Verification items for the finished model (mm, model axes). A direction names the side the tool comes from. Round coordinates to 2 decimals unless told otherwise and drop trailing zeros. Order: outer loops, then holes, each group sorted by start corner. A loop starts at its lowest first (then second) coordinate and runs counter-clockwise, first axis right, second up. Notation, with made-up numbers: M 77,23 L 118,23 A24 cw 118,34 Z; hole C 8,82 d5. An arc over 180 degrees is marked long. Return JSON: item names as keys, results as strings. Group by question number.
from build123d import *

# Parameters (mm, degrees)
SKETCH_W        = 63.5
SKETCH_H        = 21
PAD_DEPTH       = 25
SKETCH001_W     = 63
SKETCH001_H     = 21
POCKET_DEPTH    = 25
SKETCH006_W     = 8
SKETCH006_H     = 6
SKETCH006_H_2   = 2.5
POCKET004_DEPTH = 5
SKETCH007_R     = 0.7
POCKET005_DEPTH = 5
CHAMFER_SIZE    = 0.6


with BuildPart() as part:
    # Sketch → Pad (new body)
    with BuildSketch(Plane.XY):
        with Locations((31.75, 10.5)):
            Rectangle(SKETCH_W, SKETCH_H)
    extrude(amount=PAD_DEPTH)

    # Sketch001 (on Face6 of Pad) → Pocket (cut)
    with BuildSketch(Plane.XY.offset(25)):
        with Locations((32.5, 10.5)):
            Rectangle(SKETCH001_W, SKETCH001_H)
    extrude(amount=-POCKET_DEPTH, mode=Mode.SUBTRACT)

    # Sketch006 → Pocket004 (cut)
    with BuildSketch(Plane(origin=(0, 0, 0), x_dir=(0, -1, 0), z_dir=(-1, 0, 0))):
        with Locations((-10.5, 15)):
            Rectangle(SKETCH006_W, SKETCH006_H)
        with Locations((-10.5, 3.75)):
            Rectangle(SKETCH006_W, SKETCH006_H_2)
    extrude(amount=-POCKET004_DEPTH, mode=Mode.SUBTRACT)

    # Sketch007 (on Face5 of Pocket004) → Pocket005 (cut)
    with BuildSketch(Plane(origin=(0, 0, 0), x_dir=(0, -1, 0), z_dir=(-1, 0, 0))):
        with Locations((-19.5, 1.5)):
            Circle(SKETCH007_R)
        with Locations((-1.5, 1.5)):
            Circle(SKETCH007_R)
        with Locations((-1.5, 23.5)):
            Circle(SKETCH007_R)
        with Locations((-19.5, 23.5)):
            Circle(SKETCH007_R)
    extrude(amount=-POCKET005_DEPTH, mode=Mode.SUBTRACT)

    # Chamfer
    chamfer_edges = [part.edges().sort_by_distance(p)[0] for p in [
        (0, 2.2, 1.5),
        (0, 20.2, 1.5),
        (0, 20.2, 23.5),
        (0, 2.2, 23.5),
    ]]
    chamfer(chamfer_edges, length=CHAMFER_SIZE)


solid = part.part
1. Thickness scan on line 1 along Z through (x, y) = (0.75, 1.5); line 2 along Z through (x, y) = (0.15, 13.5); line 3 along Y through (x, z) = (0.9, 16.5). Record the ranges inside material, lowest first. Write a range as from..to.
2. Draft check along Z on faces 1 (the face through (0, 10, 10)), 2 (the face through (0.5, 14.5, 15)), 3 (the face through (0.5, 10.6, 25)). Enter one of: +Z half, -Z half, draft (parallel to the pull), parting line (faces both ways), or undercut.
3. Cross-section at C-C (y = 1.5). Enter the section's corners in (x, z), plus the area to 3 significant figures.
4. Access from +Z, -Z, +X, -X, +Y, -Y to the whole of each face (thin tool, end or side, straight path). Record for faces 4 (the face through (0.5, 0, 12.3)), 5 (the face through (0.5, 6.5, 15)).
5. Go/stop test with a flat-tipped pin: pin 1 (1.8 mm diameter, centred on y = 1.5, z = 1.5, fed in from -X). Record where the tip stops, or that it passes through.
6. Cross-section at D-D (y = 8.25). Enter the section's corners in (x, z), plus the area to 3 significant figures.
7. Cross-section at A-A (z = 1.5). Enter the section's corners in (x, y), plus the area to 3 significant figures.
8. Cross-section at B-B (x = 0.8). Enter the section's corners in (y, z), plus the area to 3 significant figures.
Computed:
{
 "1": {"line 1": "z = 0..0.8, 2.2..22.8, 24.2..25", "line 2": "z = 0..2.5, 5..12, 18..25", "line 3": "y = 0..6.5, 14.5..21"},
 "2": {"face 1": "draft", "face 2": "undercut", "face 3": "+Z half"},
 "3": {"outline": "M 0,0 L 1,0 L 1,0.8 L 0.6,0.8 L 0,0.2 Z; M 0,2.8 L 0.6,2.2 L 1,2.2 L 1,22.8 L 0.6,22.8 L 0,22.2 Z; M 0,24.8 L 0.6,24.2 L 1,24.2 L 1,25 L 0,25 Z", "area": "21.5 mm²"},
 "4": {"face 4": "+Z, -Z, +X, -X, -Y", "face 5": "+X, -X"},
 "5": {"pin 1": "stops at x = 0.4"},
 "6": {"outline": "M 0,0 L 1,0 L 1,2.5 L 0,2.5 Z; M 0,5 L 1,5 L 1,12 L 0,12 Z; M 0,18 L 1,18 L 1,25 L 0,25 Z", "area": "16.5 mm²"},
 "7": {"outline": "M 0,0 L 1,0 L 1,0.8 L 0.6,0.8 L 0,0.2 Z; M 0,2.8 L 0.6,2.2 L 1,2.2 L 1,18.8 L 0.6,18.8 L 0,18.2 Z; M 0,20.8 L 0.6,20.2 L 1,20.2 L 1,21 L 0,21 Z", "area": "17.5 mm²"},
 "8": {"outline": "M 0,0 L 21,0 L 21,25 L 0,25 Z; hole C 1.5,1.5 d1.4; hole C 1.5,23.5 d1.4; hole M 6.5,2.5 L 14.5,2.5 L 14.5,5 L 6.5,5 Z; hole M 6.5,12 L 14.5,12 L 14.5,18 L 6.5,18 Z; hole C 19.5,1.5 d1.4; hole C 19.5,23.5 d1.4", "area": "451 mm²"}
}
